```python
from build123d import *

# Parameters (mm, degrees)
F1_DEPTH = 60
F2_R     = 5
F3_R     = 22.203216
F4_DEPTH = 25


with BuildPart() as f1:
    # F0 (on Front) → F1 (new body)
    with BuildSketch(Plane.XZ):
        with BuildLine():
            Line((47.853137, 75.714735), (-22.146863, 75.714735))
            ThreePointArc((-22.146863, 75.714735), (-43.360067, 66.927938), (-52.146863, 45.714735))
            Line((-52.146863, 45.714735), (-52.146863, -24.285265))
            Line((-52.146863, -24.285265), (17.853137, -24.285265))
            ThreePointArc((17.853137, -24.285265), (39.06634, -15.498468), (47.853137, 5.714735))
            Line((47.853137, 5.714735), (47.853137, 75.714735))
        make_face()
    extrude(amount=F1_DEPTH)

    # F2
    f2_edges = [f1.edges().sort_by_distance(p)[0] for p in [
        (-22.146863, -30, 75.714735),
        (-52.146863, -30, 45.714735),
        (-43.360067, 0, 66.927938),
        (-43.360067, -60, 66.927938),
        (47.853137, -60, 40.714735),
        (12.853137, -60, 75.714735),
        (-52.146863, -60, 10.714735),
        (-17.146863, -60, -24.285265),
        (39.06634, -60, -15.498468),
    ]]
    fillet(f2_edges, radius=F2_R)

    # F3 (on face) → F4 (cut)
    with BuildSketch(Plane.XZ.offset(60)):
        with Locations((0, 27.350072)):
            Circle(F3_R)
    extrude(amount=-F4_DEPTH, mode=Mode.SUBTRACT)


solid = f1.part
```
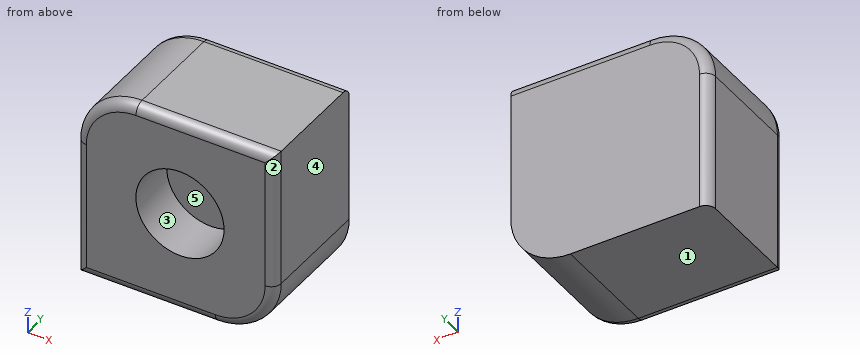
Geometry check sheet. Reference: the model listing, model coordinates, mm. Face numbers are marked on the shaded views. A direction names the side the tool comes from. Round coordinates to 2 decimals unless told otherwise and drop trailing zeros. Order: outer loops, then holes, each group sorted by start corner. A loop starts at its lowest first (then second) coordinate and runs counter-clockwise, first axis right, second up. Notation, with made-up numbers: (87.25, 23) -> (137.25, 23) arc R23 ccw to (137.25, 51) -> close; hole circle Ø1 at (-35.5, 20). An arc over 180 degrees is marked (long way). Return JSON: item names as keys, results as strings. Group by question number.
Q1. Tool access check on the marked faces 4 and 5. Record the directions out of +Z, -Z, +X, -X, +Y, -Y that give a thin tool (end or side, any length) a straight path to the whole face; none if there is none.
Q2. Section check C-C, the plane z = 43.5. Record the boundary of the cut face in (x, y), plus the area to 3 significant figures.
Q3. Material ranges on probe 1 along Z at (x, y) = (0, -48); probe 2 along Z at (x, y) = (-16, -43); probe 3 along Y at (x, z) = (4.5, 27), recorded low to high. Write a range as from..to.
Q4. Section check B-B, the plane x = 0. Record the boundary of the cut face in (y, z).
Q5. Gauge pin test, flat ends, axial feed: pin 1 (13.5 mm diameter, centred on x = 7.5, z = 26.5, fed in from -Y); pin 2 (1.5 mm diameter, centred on y = -48, z = -2, fed in from +X); pin 3 (12 mm diameter, centred on y = -15.5, z = 51, fed in from -X); pin 4 (3 mm diameter, centred on y = -50, z = 3, fed in from +X). Record the tip position at first contact, or that the pin passes through.
Q6. Section check A-A, the plane y = -48. Record the boundary of the cut face in (x, z), plus the area to 3 significant figures.
Q7. Section check D-D, the plane y = -11.5. Record the boundary of the cut face in (x, z).
Q8. Release check for a two-part mould opening along X. For the marked faces 1, 2 and 3 record: released by +X, released by -X, zero draft, split by the parting line, or undercut.
Numbers:
{
 "1": {"face 4": "+Z, -Z, +X, +Y, -Y", "face 5": "-Y"},
 "2": {"outline": "(-52.15, -55) arc R5 ccw to (-47.15, -60) -> (-15.24, -60) -> (-15.24, -35) -> (15.24, -35) -> (15.24, -60) -> (42.85, -60) arc R5 ccw to (47.85, -55) -> (47.85, 0) -> (-47.15, 0) arc R5 ccw to (-52.15, -5) -> close", "area": "5,220 mm^2"},
 "3": {"probe 1": "-24.29..5.15, 49.55..75.71", "probe 2": "-24.29..11.96, 42.74..75.71", "probe 3": "-35..0"},
 "4": {"outline": "(-60, -19.29) arc R5 ccw to (-55, -24.29) -> (0, -24.29) -> (0, 70.71) arc R5 ccw to (-5, 75.71) -> (-55, 75.71) arc R5 ccw to (-60, 70.71) -> (-60, 49.55) -> (-35, 49.55) -> (-35, 5.15) -> (-60, 5.15) -> close"},
 "5": {"pin 1": "y = -35", "pin 2": "x = 47.03", "pin 3": "x = -52.15", "pin 4": "x = 47.83"},
 "6": {"outline": "(-52.15, -24.29) -> (17.85, -24.29) arc R30 ccw to (47.85, 5.71) -> (47.85, 75.71) -> (-22.15, 75.71) arc R30 ccw to (-52.15, 45.71) -> close; hole circle Ø44.41 at (0, 27.35)", "area": "8,060 mm^2"},
 "7": {"outline": "(-52.15, -24.29) -> (17.85, -24.29) arc R30 ccw to (47.85, 5.71) -> (47.85, 75.71) -> (-22.15, 75.71) arc R30 ccw to (-52.15, 45.71) -> close"},
 "8": {"face 1": "zero draft", "face 2": "released by +X", "face 3": "undercut"}
}
